from build123d import *

# Parameters (mm, degrees)
PAD_DEPTH       = 3.5
SKETCH001_R     = 2.7
POCKET_DEPTH    = 5
SKETCH002_R     = 20
POCKET001_DEPTH = 5


with BuildPart() as part:
    # Sketch → Pad (new body)
    with BuildSketch(Plane.XY):
        Polygon((0, 0), (40, 0), (40, 20), (20, 40), (0, 40), align=None)
    extrude(amount=PAD_DEPTH)

    # Sketch001 → Pocket (cut)
    with BuildSketch(Plane.XY.offset(3.5)):
        with Locations((9, 29)):
            Circle(SKETCH001_R)
        with Locations((29, 9)):
            Circle(SKETCH001_R)
        with Locations((9, 9)):
            Circle(SKETCH001_R)
    extrude(amount=-POCKET_DEPTH, mode=Mode.SUBTRACT)

    # Sketch002 → Pocket001 (cut)
    with BuildSketch(Plane.XY.offset(3.5)):
        with Locations((40, 40)):
            Circle(SKETCH002_R)
    extrude(amount=-POCKET001_DEPTH, mode=Mode.SUBTRACT)


solid = part.part
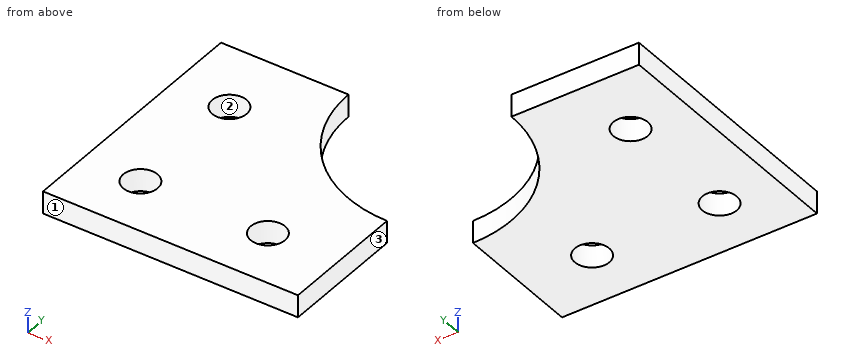
Design review of the part built by this model. Coordinates are the model's own, in mm. Face numbers are marked on the shaded views. Give positions to 0.01 mm unless a question says otherwise; leave off trailing zeros. Write each loop counter-clockwise with the first axis right and the second up, starting at its lowest first coordinate (ties: lowest second). Pieces come first, ordered by that corner, then holes. Notation, with made-up numbers: M -16.5,75.25 L 28.5,75.25 A20 ccw 28.5,97.25 Z; hole C 31,69 d9. An arc over 180 degrees is marked long. Answer as a JSON object with one key per item and string values. Group by question number.
1) Clearance check with a flat-ended pin moving along its axis: pin 1 Ø5 at (x, y) = (9, 29) entering from -Z. State where the tip first meets the part, or that it passes through.
2) We need section D-D (y = 29). Give the boundary of the cut face in (x, z), and give its area (3 significant figures).
3) We need section B-B (z = 1.2). Give the boundary of the cut face in (x, y), and give its area (3 significant figures).
4) For line 1 along Y through (x, z) = (9, 1.95); line 2 along X through (y, z) = (27, 0.95); line 3 along X through (y, z) = (7.5, 0.4) (3 decimals), list the stretches that pass through material, from the lowest coordinate up.
5) Mouldability with a two-part tool opening along Y and no side actions: class the marked faces 1, 2 and 3 as released by +Y, released by -Y, zero draft, split by the parting line, or undercut.
6) We need section A-A (x = 9). Give the boundary of the cut face in (y, z), and give its area (3 significant figures).
Answer key:
{
 "1": {"pin 1": "passes through"},
 "2": {"outline": "M 0,0 L 6.3,0 L 6.3,3.5 L 0,3.5 Z; M 11.7,0 L 23.3,0 L 23.3,3.5 L 11.7,3.5 Z", "area": "62.6 mm²"},
 "3": {"outline": "M 0,0 L 40,0 L 40,20 A20 cw 20,40 L 0,40 Z; hole C 9,9 d5.4; hole C 9,29 d5.4; hole C 29,9 d5.4", "area": "1,220 mm²"},
 "4": {"line 1": "y = 0 to 6.3, 11.7 to 26.3, 31.7 to 40", "line 2": "x = 0 to 7.19, 10.81 to 24.8", "line 3": "x = 0 to 6.755, 11.245 to 26.755, 31.245 to 40"},
 "5": {"face 1": "released by -Y", "face 2": "undercut", "face 3": "zero draft"},
 "6": {"outline": "M 0,0 L 6.3,0 L 6.3,3.5 L 0,3.5 Z; M 11.7,0 L 26.3,0 L 26.3,3.5 L 11.7,3.5 Z; M 31.7,0 L 40,0 L 40,3.5 L 31.7,3.5 Z", "area": "102 mm²"}
}
